Read the model definition and answer for the solid it produces. Units are mm, in the model's axes. A direction names the side the tool comes from. Coordinates: 2 decimals unless noted, no trailing zeros. Order: outer loops, then holes, each group sorted by start corner. A loop starts at its lowest first (then second) coordinate and runs counter-clockwise, first axis right, second up. Notation, with made-up numbers: M -4.75,14.25 L 6.25,14.25 A18 cw 6.25,38.25 Z; hole C -35,65 d4. An arc over 180 degrees is marked long. Put each result on its own line as item: value.
from build123d import *

# Parameters (mm, degrees)
ESBO_O1_W                  = 200
ESBO_O1_H                  = 178
RESSALTO_EXTRUS_O1_DEPTH   = 10
ESBO_O3_W                  = 200
ESBO_O3_H                  = 10
RESSALTO_EXTRUS_O2_DEPTH   = 150
CORTE_EXTRUS_O1_DEPTH      = 346.594052101
CORTE_EXTRUS_O1_DEPTH_BACK = 346.594052101
ESBO_O4_R                  = 5


with BuildPart() as part:
    # Esboço1 → Ressalto-extrusão1 (new body)
    with BuildSketch(Plane.XY):
        with Locations((-198.352557971, 0)):
            Rectangle(ESBO_O1_W, ESBO_O1_H)
    extrude(amount=RESSALTO_EXTRUS_O1_DEPTH)

    # Esboço3 → Ressalto-extrusão2 (add)
    with BuildSketch(Plane.XY.offset(10)):
        with Locations((-198.352557971, 84)):
            Rectangle(ESBO_O3_W, ESBO_O3_H)
    extrude(amount=RESSALTO_EXTRUS_O2_DEPTH)

    # Esboço4 → Corte-extrusão1 (cut, two sides: drawn at the far end of the back side and taken through both)
    with BuildSketch(Plane.XY.offset(10).offset(-CORTE_EXTRUS_O1_DEPTH_BACK)):
        with Locations((-231.685557971, -0.1112)):
            Circle(ESBO_O4_R)
    extrude(amount=CORTE_EXTRUS_O1_DEPTH + CORTE_EXTRUS_O1_DEPTH_BACK, mode=Mode.SUBTRACT)


solid = part.part
Q1. A tool of negligible diameter and unlimited length cuts with its end or side. For faces 1 (the face through (-200, 79, 84)), 2 (the face through (-298.353, 26, 9)), from which of +Z, -Z, +X, -X, +Y, -Y can it reach the whole face along a straight path? Write none if from no direction.
Answers below:
face 1: +Z, +X, -X, -Y
face 2: +Z, -Z, -X, +Y, -Y
Q2. Find section A-A on x = -230. Write down the section's boundary in (y, z), plus the area to 3 significant figures.
Answers below:
outline: M -89,0 L -4.82,0 L -4.82,10 L -89,10 Z; M 4.6,0 L 89,0 L 89,160 L 79,160 L 79,10 L 4.6,10 Z
area: 3,190 mm^2
Q3. Find section C-C on z = 135. Write down the section's boundary in (x, y).
Answers below:
outline: M -298.35,79 L -98.35,79 L -98.35,89 L -298.35,89 Z
Q4. Find section B-B on y = 60.5. Write down the section's boundary in (x, z).
Answers below:
outline: M -298.35,0 L -98.35,0 L -98.35,10 L -298.35,10 Z
Q5. Given pin 1 (8 mm diameter, centred on x = -208.5, z = 24.5, fed in from -Y); pin 2 (6 mm diameter, centred on x = -201.5, y = 37.5, fed in from +Z), each flat-ended and moving along its own axis, determine where each tip first touches the part or whether it passes through.
Answers below:
pin 1: stops at y = 79
pin 2: stops at z = 10
Q6. Find section D-D on x = -251. Write down the section's boundary in (y, z).
Answers below:
outline: M -89,0 L 89,0 L 89,160 L 79,160 L 79,10 L -89,10 Z
Q7. Consider line 1 along Z through (x, y) = (-272, -36); line 2 along Y through (x, z) = (-177.5, 88). Determine where each line is inside the solid, lowest interval first.
Answers below:
line 1: z = 0 to 10
line 2: y = 79 to 89
